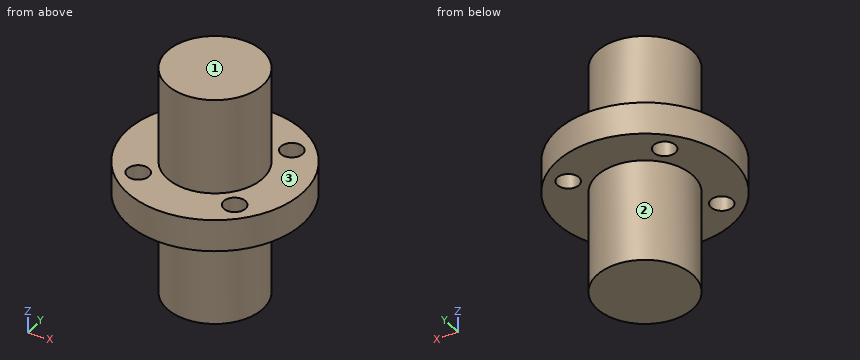
from build123d import *

# Parameters (mm, degrees)
SKETCH_1_R           = 27.5
SKETCH_1_R_2         = 3
EXTRUDE_1_DEPTH      = 10
HOLE_WIZARD_M8_1_D   = 6.8
EXTRUDE_2_DEPTH      = 32
EXTRUDE_2_DEPTH_BACK = 40
SKETCH_6_R           = 15


with BuildPart() as part:
    # 草图1 → 凸台-拉伸1 (new body)
    with BuildSketch(Plane.XY):
        Circle(SKETCH_1_R)
        with Locations((-14.849242405, -14.849242405)):
            Circle(SKETCH_1_R_2, mode=Mode.SUBTRACT)
        with Locations((14.849242405, -14.849242405)):
            Circle(SKETCH_1_R_2, mode=Mode.SUBTRACT)
        with Locations((14.849242405, 14.849242405)):
            Circle(SKETCH_1_R_2, mode=Mode.SUBTRACT)
        with Locations((-14.849242405, 14.849242405)):
            Circle(SKETCH_1_R_2, mode=Mode.SUBTRACT)
    extrude(amount=EXTRUDE_1_DEPTH)

    # M8 螺纹孔1 (through all)
    with Locations(Plane(origin=(0, 0, 0), x_dir=(1, 0, 0), z_dir=(0, 0, -1))):
        with Locations((-14.849242405, -14.849242405), (14.849242405, -14.849242405), (14.849242405, 14.849242405), (-14.849242405, 14.849242405)):
            Hole(HOLE_WIZARD_M8_1_D / 2)

    # 草图6 → 凸台-拉伸2 (add, two sides: drawn at the far end of the back side and taken through both)
    with BuildSketch(Plane(origin=(0, 0, 0), x_dir=(-1, 0, 0), z_dir=(0, 0, -1)).offset(-EXTRUDE_2_DEPTH_BACK)):
        Circle(SKETCH_6_R)
    extrude(amount=EXTRUDE_2_DEPTH + EXTRUDE_2_DEPTH_BACK)


solid = part.part
The model under review builds one solid part; all positions refer to its coordinate system, in mm. Face numbers are marked on the shaded views. A direction names the side the tool comes from. Round coordinates to 2 decimals unless told otherwise and drop trailing zeros. Loops run counter-clockwise (first coordinate to the right, second up) from the corner with the lowest first, then second, coordinate; pieces in that order, holes last. Notation, with made-up numbers: M -20.75,15.5 L 13.25,15.5 A15 ccw 13.25,24.5 Z; hole C 5.5,65 d1. An arc over 180 degrees is marked long. Answer as CSV lines item,"result". Start each with the question number.
Item 1: Consider section D-D (z = -27). Write out the cut boundary in (x, y), then the cut area to 3 significant figures.
Item 2: Wall thickness on line 1 (X direction, y = -14, z = 7.5); line 2 (Z direction, x = -13, y = 9); line 3 (X direction, y = 24, z = 4.5): over which ranges is each line inside the solid? List them lowest first. Write a range as [from, to].
Item 3: For the marked faces 1, 2 and 3, list the 3-axis set-ups (+Z, -Z, +X, -X, +Y, -Y) from which the entire face can be reached by the end or side of a thin tool; tool diameter is ignored.
Item 4: Consider section A-A (y = 0). Write out the cut boundary in (x, z).
Item 5: Consider section B-B (z = 5). Write out the cut boundary in (x, y).
Item 6: Insertion check: P1, Ø1.5, axis at x = 14.5, z = 7.5, coming from the -Y side; P2, Ø6, axis at x = -10.5, z = 21.5, coming from the -Y side; P3, Ø11, axis at x = -14.85, y = 14.85, coming from the -Z side. Each pin has a flat end and moves straight along its axis. Give the tip position at first contact, or say it passes through.
Answer:
1,outline,"C 0,0 d30"
1,area,"707 mm^2"
2,line 1,"x = [-23.67, -18.14], [-11.56, 11.56], [18.14, 23.67]"
2,line 2,"z = [0, 10]"
2,line 3,"x = [-13.43, 13.43]"
3,face 1,"+Z, +X, -X, +Y, -Y"
3,face 2,"-Z"
3,face 3,"+Z"
4,outline,"M -27.5,0 L -15,0 L -15,-32 L 15,-32 L 15,0 L 27.5,0 L 27.5,10 L 15,10 L 15,40 L -15,40 L -15,10 L -27.5,10 Z"
5,outline,"C 0,0 d55; hole C -14.85,-14.85 d6.8; hole C -14.85,14.85 d6.8; hole C 14.85,-14.85 d6.8; hole C 14.85,14.85 d6.8"
6,P1,"stops at y = -23.82"
6,P2,"stops at y = -12.99"
6,P3,"stops at z = 0"
